from build123d import *

# Parameters (mm, degrees)
SKETCH1_R           = 2.38125
BOSS_EXTRUDE1_DEPTH = 6.35
FILLET1_R           = 2.38125
SKETCH2_R           = 1.5875
CUT_EXTRUDE1_DEPTH  = 26.010828999
CIRPATTERN1_COUNT   = 3


with BuildPart() as part:
    # Sketch1 → Boss-Extrude1 (new body)
    with BuildSketch(Plane.XY):
        with BuildLine():
            Line((0, 0), (19.05, 0))
            Line((19.05, 0), (19.05, 3.175))
            Line((19.05, 3.175), (12.454412895, 3.175))
            ThreePointArc((12.454412895, 3.175), (7.14375, 12.373337957), (-3.477575791, 12.373337957))
            Line((-3.477575791, 12.373337957), (-6.775369343, 18.085283942))
            Line((-6.775369343, 18.085283942), (-9.525, 16.497783942))
            Line((-9.525, 16.497783942), (0, 0))
        make_face()
        with Locations((3.571875, 6.186668978)):
            Circle(SKETCH1_R, mode=Mode.SUBTRACT)
    extrude(amount=BOSS_EXTRUDE1_DEPTH)

    # Fillet1
    fillet1_edges = [part.edges().sort_by_distance(p)[0] for p in [
        (-3.477575791, 12.373337957, 3.175),
        (12.454412895, 3.175, 3.175),
        (0, 0, 3.175),
    ]]
    fillet(fillet1_edges, radius=FILLET1_R)

    # Sketch2 → Cut-Extrude1 (cut, through all)
    with BuildSketch(Plane(origin=(0, 3.175, 0), x_dir=(1, 0, 0), z_dir=(0, 1, 0))):
        with Locations(Location((16.83287803, -3.175, 0), (0, 0, 180))):
            Circle(SKETCH2_R)
    cut_extrude1 = extrude(amount=-CUT_EXTRUDE1_DEPTH, mode=Mode.SUBTRACT)

    # CirPattern1: Cut-Extrude1 ×3 about axis
    cirpattern1_axis = Axis((0, 0, -80.9), (0, 0, 1))
    for i in range(1, CIRPATTERN1_COUNT):
        add(cut_extrude1.rotate(cirpattern1_axis, i * 360 / CIRPATTERN1_COUNT), mode=Mode.SUBTRACT)


solid = part.part
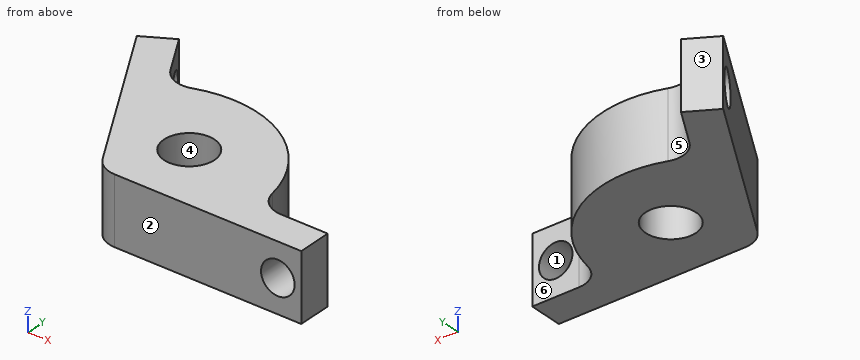
Can you work these out from the model? Positions are in its coordinate system, mm. Face numbers are marked on the shaded views. A direction names the side the tool comes from. Coordinates: 2 decimals unless noted, no trailing zeros. Loops run counter-clockwise (first coordinate to the right, second up) from the corner with the lowest first, then second, coordinate; pieces in that order, holes last. Notation, with made-up numbers: M 87.5,-6.5 L 102.5,-6.5 A17 ccw 102.5,6.5 Z; hole C 3,32.5 d3. An arc over 180 degrees is marked long. Return JSON: item names as keys, results as strings. Group by question number.
Item 1: Thinking about a two-plate mould opening in Y: for the marked faces 1, 2, 3 and 4, which applies, released by +Y, released by -Y, zero draft, split by the parting line, or undercut?
Item 2: Imagine slicing it at A-A (z = 2.25). Give the number of separate pieces and of enclosed holes in the cut face, and give its area (3 significant figures).
Item 3: If I drill on L1, parallel to Y at x = 2.5, z = 1.75; L2, parallel to X at y = 4.25, z = 5.5; L3, parallel to X at y = 1.5, z = 4.25, over which ranges is the centre line in solid material (lowest first)? Write a range as from..to.
Item 4: I'm going to push a flat-ended pin straight in: pin 1 Ø2 at (y, z) = (8.5, 4.5) entering from +X. Where does the tip first touch, or does it pass through?
Item 5: Imagine slicing it at C-C (y = 5.5). Please give me the cut outline in (x, z).
Item 6: Imagine slicing it at B-B (x = 17). Please give me the cut outline in (y, z) (3 decimals).
Item 7: On a 3-axis mill with a long thin cutter (end or side, diameter ignored), from which of +Z, -Z, +X, -X, +Y, -Y can I reach the whole of each face in a straight line? I mean the marked faces 5 and 6. Say none if no direction works.
Verdict:
{
 "1": {"face 1": "zero draft", "face 2": "released by -Y", "face 3": "released by +Y", "face 4": "undercut"},
 "2": {"separate pieces": "3", "enclosed holes": "1", "area": "201 mm^2"},
 "3": {"L1": "y = 0..4.06, 8.31..13.78", "L2": "x = -2.45..2.19, 4.96..12.62", "L3": "x = -0.87..15.66, 18..19.05"},
 "4": {"pin 1": "stops at x = 11.53"},
 "5": {"outline": "M -3.18,0 L 1.29,0 L 1.29,6.35 L -3.18,6.35 Z; M 5.85,0 L 12.2,0 L 12.2,6.35 L 5.85,6.35 Z"},
 "6": {"outline": "M 0,0 L 3.175,0 L 3.175,1.596 L 0,1.596 Z; M 0,4.754 L 3.175,4.754 L 3.175,6.35 L 0,6.35 Z"},
 "7": {"face 5": "+Z, -Z, +Y", "face 6": "+Z, -Z, +X, +Y"}
}
